from build123d import *

# Parameters (mm, degrees)
F0_W     = 127
F0_H     = 76.2
F1_DEPTH = 25.4
F2_W     = 127
F2_H     = 31.75
F3_DEPTH = 15.875
F4_R     = 6.35
F5_DEPTH = 25.401


with BuildPart() as f1:
    # F0 (on Top) → F1 (new body)
    with BuildSketch(Plane.XY):
        Rectangle(F0_W, F0_H)
    extrude(amount=F1_DEPTH)

    # F2 (on face) → F3 (cut)
    with BuildSketch(Plane(origin=(0, 0, 0), x_dir=(1, 0, 0), z_dir=(0, 0, -1))):
        Rectangle(F2_W, F2_H)
    extrude(amount=-F3_DEPTH, mode=Mode.SUBTRACT)

    # F4 (on face) → F5 (cut, through all)
    with BuildSketch(Plane.XY.offset(25.4)):
        with Locations((25.4, 28.575)):
            Circle(F4_R)
        with Locations((25.4, -28.575)):
            Circle(F4_R)
    extrude(amount=-F5_DEPTH, mode=Mode.SUBTRACT)


solid = f1.part
For this review, take the finished solid that the model builds, in its own axes (mm). A direction names the side the tool comes from. Give positions to 0.01 mm unless a question says otherwise; leave off trailing zeros. Write each loop counter-clockwise with the first axis right and the second up, starting at its lowest first coordinate (ties: lowest second). Pieces come first, ordered by that corner, then holes. Notation, with made-up numbers: (20, 69.25) -> (41, 69.25) arc R11 cw to (41, 89.25) -> close; hole circle Ø2 at (69.25, 18.5). An arc over 180 degrees is marked (long way). Use CSV: the item, a comma, the result in double quotes.
Q1. Tool access review of faces 1 (the face through (-1, 38.1, 13)), 2 (the face through (-1, 0, 15.875)): name each direction out of +Z, -Z, +X, -X, +Y, -Y from which nothing blocks a thin tool from reaching the whole face with its end or side.
Conclusion:
face 1,"+Z, -Z, +X, -X, +Y"
face 2,"-Z, +X, -X"
Q2. Take a section at C-C, the plane z = 21.75. Write out the cut boundary in (x, y) (3 decimals).
Conclusion:
outline,"(-63.5, -38.1) -> (63.5, -38.1) -> (63.5, 38.1) -> (-63.5, 38.1) -> close; hole circle Ø12.7 at (25.4, -28.575); hole circle Ø12.7 at (25.4, 28.575)"
Q3. For P1, Ø9.5, axis at x = -18.5, y = 4.5, coming from the -Z side (3 decimals), flat-tipped, find the tip position at first contact; note if it passes through.
Conclusion:
P1,"z = 15.875"
Q4. To check wall thickness, follow probe 1 along Y at (x, z) = (25.4, 20) (3 decimals); probe 2 along Y at (x, z) = (25.4, 11.25) (3 decimals); probe 3 along Y at (x, z) = (21, 12) (3 decimals). State the ranges of each line that lie inside material, in increasing order. Write a range as [from, to].
Conclusion:
probe 1,"[-38.1, -34.925], [-22.225, 22.225], [34.925, 38.1]"
probe 2,"[-38.1, -34.925], [-22.225, -15.875], [15.875, 22.225], [34.925, 38.1]"
probe 3,"[-38.1, -33.153], [-23.997, -15.875], [15.875, 23.997], [33.153, 38.1]"
Q5. Take a section at A-A, the plane x = 25.4. Write out the cut boundary in (y, z) (3 decimals).
Conclusion:
outline,"(-38.1, 0) -> (-34.925, 0) -> (-34.925, 25.4) -> (-38.1, 25.4) -> close; (-22.225, 0) -> (-15.875, 0) -> (-15.875, 15.875) -> (15.875, 15.875) -> (15.875, 0) -> (22.225, 0) -> (22.225, 25.4) -> (-22.225, 25.4) -> close; (34.925, 0) -> (38.1, 0) -> (38.1, 25.4) -> (34.925, 25.4) -> close"
Q6. Mouldability with a two-part tool opening along Y and no side actions: class faces 3 (the face through (24.57, -22.28, 12.88)), 4 (the face through (-1, -27, 0)), 5 (the face through (-1, -38.1, 13)), 6 (the face through (24.023, 22.376, 12.878)) as pulls with the +Y half, pulls with the -Y half, needs draft (parallel to the pull), parting line crosses it, or undercut.
Conclusion:
face 3,"undercut"
face 4,"needs draft"
face 5,"pulls with the -Y half"
face 6,"undercut"
Q7. Take a section at B-B, the plane z = 6.5. Write out the cut boundary in (x, y) (3 decimals), then the cut area to 3 significant figures.
Conclusion:
outline,"(-63.5, -38.1) -> (63.5, -38.1) -> (63.5, -15.875) -> (-63.5, -15.875) -> close; (-63.5, 15.875) -> (63.5, 15.875) -> (63.5, 38.1) -> (-63.5, 38.1) -> close; hole circle Ø12.7 at (25.4, -28.575); hole circle Ø12.7 at (25.4, 28.575)"
area,"5,390 mm2"
